from build123d import *

# Parameters (mm, degrees)
F0_W     = 50
F0_H     = 220
F1_DEPTH = 30
F2_W     = 200.0000000022
F2_H     = 10
F3_DEPTH = 50
F5_DEPTH = 220
F6_DEPTH = 25
F7_R     = 3.75
F8_DEPTH = 10


with BuildPart() as f1:
    # F0 (on Top) → F1 (new body)
    with BuildSketch(Plane.XY):
        with Locations((-38.1634101286, 8.3829769865)):
            Rectangle(F0_W, F0_H)
    extrude(amount=F1_DEPTH)

    # F2 (on face) → F3 (cut, through all)
    with BuildSketch(Plane.YZ.offset(-13.1634101286)):
        with Locations((8.3829769876, 15)):
            Rectangle(F2_W, F2_H)
    extrude(amount=-F3_DEPTH, mode=Mode.SUBTRACT)

    # F4 (on face) → F5 (cut, through all)
    with BuildSketch(Plane.XZ.offset(101.6170230135)):
        Polygon((-63.1634101286, 30), (-63.1634101286, 20.3228145838), (-23.2081543654, 30), align=None)
    extrude(amount=-F5_DEPTH, mode=Mode.SUBTRACT)

    # F6 (add): a face of the model
    f6_faces = [f1.faces().sort_by_distance(p)[0] for p in [
        (-18.185782247, 8.3829769865, 30),
    ]]
    extrude(f6_faces, amount=F6_DEPTH)

    # F7 (on face) → F8 (join)
    with BuildSketch(Plane(origin=(0, 0, 0), x_dir=(1, 0, 0), z_dir=(0, 0, -1))):
        with Locations((-56.7856021225, -108.2918941975)):
            Circle(F7_R)
        with Locations((-56.7856021225, -83.2918941975)):
            Circle(F7_R)
        with Locations((-56.7856021225, -58.2918941975)):
            Circle(F7_R)
        with Locations((-56.7856021225, -33.2918941975)):
            Circle(F7_R)
        with Locations((-56.7856021225, -8.2918941975)):
            Circle(F7_R)
        with Locations((-56.7856021225, 16.7081058025)):
            Circle(F7_R)
        with Locations((-56.7856021225, 41.7081058025)):
            Circle(F7_R)
        with Locations((-56.7856021225, 66.7081058025)):
            Circle(F7_R)
        with Locations((-56.7856021225, 91.7081058025)):
            Circle(F7_R)
    extrude(amount=F8_DEPTH)


solid = f1.part
Work out the finished part from the listing and answer in its coordinate system (mm). A direction names the side the tool comes from. Round coordinates to 2 decimals unless told otherwise and drop trailing zeros. Order: outer loops, then holes, each group sorted by start corner. A loop starts at its lowest first (then second) coordinate and runs counter-clockwise, first axis right, second up. Notation, with made-up numbers: M -13,-28 L 27,-28 A19 ccw 27,-17 Z; hole C 43,52 d10. An arc over 180 degrees is marked long. Put each result on its own line as item: value. Start each with the question number.
Q1. Section D-D, the plane x = -31.5 is taken. Write down the section's boundary in (y, z), and give its area (3 significant figures).
Q2. For a pull along Y with two mould halves and no side action, classify faces 4 (the cylindrical face through (-57.599, 61.953, -4.93)), 5 (the cylindrical face through (-60.532, -16.873, -4.93)), 6 (the flat face through (-57, 58, -10)), 7 (the flat face through (-33, -101.617, 21)) as pulls with the +Y half, pulls with the -Y half, needs draft (parallel to the pull), parting line crosses it, or undercut.
Q3. Flat-ended cylindrical pins translate along their axes: pin 1 (8 mm diameter, centred on x = -37, y = -42, fed in from -Z); pin 2 (6 mm diameter, centred on x = -32, y = 92.5, fed in from +Z); pin 3 (2 mm diameter, centred on x = -43.5, z = 27, fed in from +Y). Find the tip coordinate at first contact, or state that the pin passes through.
Q4. Section A-A, the plane y = 70 is taken. Write down the section's boundary in (x, z), and give its area (3 significant figures).
Q5. A tool of negligible diameter and unlimited length cuts with its end or side. For faces 1 (the cylindrical face through (-59.55, 105.76, -4.93)), 2 (the flat face through (-38, 7, 20)), 3 (the flat face through (-33, 118.383, 21)), from which of +Z, -Z, +X, -X, +Y, -Y can it reach the whole face along a straight path? Write none if from no direction.
Q6. Section B-B, the plane z = 15 is taken. Write down the section's boundary in (x, y).
Q7. Section C-C, the plane z = -3 is taken. Give the number of separate pieces and of enclosed holes in the cut face, and give its area (3 significant figures).
Q8. Straight lines are drawn through the part: L1, parallel to Z at x = -21, y = -27; L2, parallel to Y at x = -27.5, z = 19.5; L3, parallel to X at y = 104, z = 42. For each, find the intervals that lie inside material, in ascending order. Write a range as [from, to].
Findings below:
1. outline: M -101.62,0 L 118.38,0 L 118.38,27.99 L -101.62,27.99 Z; hole M -91.62,10 L 108.38,10 L 108.38,20 L -91.62,20 Z
1. area: 4,160 mm^2
2. face 4: undercut
2. face 5: undercut
2. face 6: needs draft
2. face 7: pulls with the -Y half
3. pin 1: stops at z = 0
3. pin 2: stops at z = 28.6
3. pin 3: passes through
4. outline: M -63.16,0 L -13.16,0 L -13.16,10 L -63.16,10 Z; M -63.16,20 L -13.16,20 L -13.16,55 L -23.21,55 L -23.21,30 L -63.16,20.32 Z
4. area: 1,060 mm^2
5. face 1: -Z
5. face 2: +X, -X
5. face 3: +Z, -Z, +X, -X, +Y
6. outline: M -63.16,-101.62 L -13.16,-101.62 L -13.16,-91.62 L -63.16,-91.62 Z; M -63.16,108.38 L -13.16,108.38 L -13.16,118.38 L -63.16,118.38 Z
7. separate pieces: 9
7. enclosed holes: 0
7. area: 398 mm^2
8. L1: z = [0, 10], [20, 55]
8. L2: y = [-101.62, -91.62], [108.38, 118.38]
8. L3: x = [-23.21, -13.16]
